Can you work these out from the model? Positions are in its coordinate system, mm. A direction names the side the tool comes from. Give positions to 0.01 mm unless a question says otherwise; leave off trailing zeros. Loops run counter-clockwise (first coordinate to the right, second up) from the corner with the lowest first, then second, coordinate; pieces in that order, holes last. Notation, with made-up numbers: (35.5, 47.25) - (47.5, 47.25) arc R18 cw to (47.5, 63.25) - close; hole circle Ø5 at (80.25, 15.5). An arc over 180 degrees is marked (long way). Answer as a JSON object with one key per item and string values.
```python
from build123d import *

# Parameters (mm, degrees)
F0_R     = 25.032826
F2_DEPTH = 14.944287
F1_R     = 21.08274
F3_DEPTH = 20.706544
F5_DEPTH = 25.4


with BuildPart() as f2:
    # F0 (on Top) → F2 (new body)
    with BuildSketch(Plane.XY):
        Circle(F0_R)
    extrude(amount=F2_DEPTH)

    # F1 (on face) → F3 (cut)
    with BuildSketch(Plane.XY):
        Circle(F1_R)
    extrude(amount=F3_DEPTH, mode=Mode.SUBTRACT)

    # F4 (on Front) → F5 (cut)
    with BuildSketch(Plane.XZ):
        Polygon((-8.591931, 10.888215), (-13.923068, 6.954562), (-11.59393, 7.161595), (-8.229621, 8.248527), (-4.865311, 9.490732), (0.465825, 9.024907), (5.362451, 9.060643), (10.972824, 7.368632), (11.956234, 10.629423), (1.915064, 10.888215), align=None)
    extrude(amount=F5_DEPTH, mode=Mode.SUBTRACT)


solid = f2.part
```
1) Imagine slicing it at B-B on x = 4. Write out the boundary of the cut face in (y, z), and give its area (3 significant figures).
Check sheet entries:
{"outline": "(-24.71, 0) - (-20.7, 0) - (-20.7, 9.05) - (-24.71, 9.05) - close; (-24.71, 10.83) - (-20.7, 10.83) - (-20.7, 14.94) - (-24.71, 14.94) - close; (20.7, 0) - (24.71, 0) - (24.71, 14.94) - (20.7, 14.94) - close", "area": "113 mm2"}
2) I need wall thicknesses on L1, parallel to Y at x = 0, z = 6.5; L2, parallel to Y at x = -8.5, z = 1.75; L3, parallel to X at y = 5, z = 10. Which ranges of each line are inside material? Lowest first, please.
Check sheet entries:
{"L1": "-25.03 to -21.08, 21.08 to 25.03", "L2": "-23.55 to -19.29, 19.29 to 23.55", "L3": "-24.53 to -20.48, 20.48 to 24.53"}
3) Imagine slicing it at C-C on z = 13.5. Write out the boundary of the cut face in (x, y), and give its area (3 significant figures).
Check sheet entries:
{"outline": "circle Ø50.07 at (0, 0); hole circle Ø42.17 at (0, 0)", "area": "572 mm2"}
4) I'm going to push flat-ended pins straight in: P1, Ø5, axis at x = -0.5, z = 12.5, coming from the +Y side; P2, Ø1, axis at x = 4, z = 3, coming from the +Y side. Where does each tip first touch, or does it pass through?
Check sheet entries:
{"P1": "y = 25.03", "P2": "y = 24.79"}
5) Imagine slicing it at D-D on y = 14. Write out the boundary of the cut face in (x, z), and give its area (3 significant figures).
Check sheet entries:
{"outline": "(-20.75, 0) - (-15.76, 0) - (-15.76, 14.94) - (-20.75, 14.94) - close; (15.76, 0) - (20.75, 0) - (20.75, 14.94) - (15.76, 14.94) - close", "area": "149 mm2"}
6) If we mould it in two halves opening along X, with no side actions, what happens to faces 1 (the flat face through (-13, -17, 0)), 2 (the flat face through (-9.935, -20.583, 7.697)), 3 (the cylindrical face through (13.457, 21.108, 7.368))? For each: released by +X, released by -X, zero draft, split by the parting line, or undercut.
Check sheet entries:
{"face 1": "zero draft", "face 2": "undercut", "face 3": "split by the parting line"}
7) Which directions (+Z, -Z, +X, -X, +Y, -Y) give clear straight access to the entire face, cutting with the end or side of a thin tool? Please do faces 4 (the flat face through (-13, -17, 14.944)), 5 (the flat face through (-3, -23, 10.888)).
Check sheet entries:
{"face 4": "+Z, +X, -X, +Y, -Y", "face 5": "-Y"}
8) Imagine slicing it at A-A on y = -2. Write out the boundary of the cut face in (x, z).
Check sheet entries:
{"outline": "(-24.95, 0) - (-20.99, 0) - (-20.99, 14.94) - (-24.95, 14.94) - close; (20.99, 0) - (24.95, 0) - (24.95, 14.94) - (20.99, 14.94) - close"}
